Geometry: see drawing. Coordinates: mm, zero at the bounding-box minimum. Give positions to 0.01 mm unless a question says otherwise; leave off trailing zeros. Loops run counter-clockwise (first coordinate to the right, second up) from the corner with the lowest first, then second, coordinate; pieces in that order, holes last. Notation, with made-up numbers: (21.25, 67) - (70.25, 67) arc R17 ccw to (70.25, 73) - close; hole circle Ø8 at (35.5, -31). An arc over 180 degrees is marked (long way). Use one line per item in the form item = value.
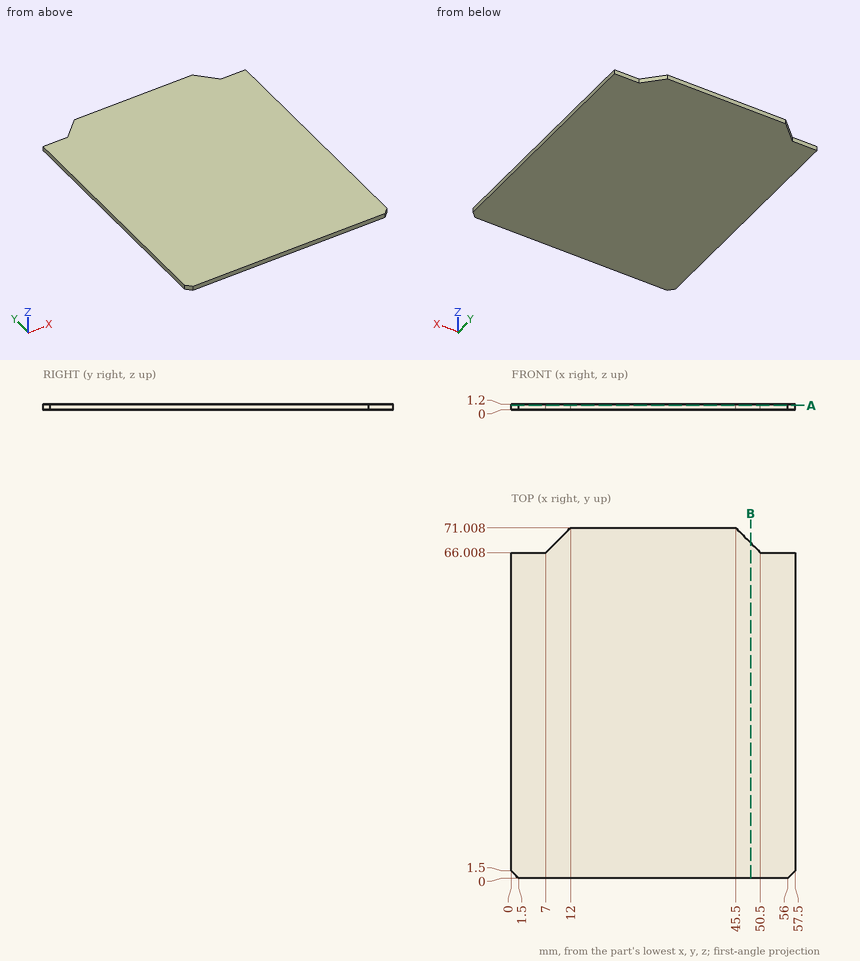
(1) Pin query (flat end, axial travel): P1, Ø0.6, axis at x = 3.5, z = 1, coming from the +Y side. Return the tip coordinate at first contact, or that it passes through.
Solution:
P1 = 66.01
(2) Material intervals for L1, parallel to Y at x = 6, z = 0.2; L2, parallel to Y at x = 11.5, z = 0.7, sorted ascending. Write a range as from..to.
Solution:
L1 = 0..66.01
L2 = 0..70.51
(3) Cut plane A-A (z = 0.9). Return the cut outline in (x, y), plus the area to 3 significant figures.
Solution:
outline = (0, 1.5) - (1.5, 0) - (56, 0) - (57.5, 1.5) - (57.5, 66.01) - (50.5, 66.01) - (45.5, 71.01) - (12, 71.01) - (7, 66.01) - (0, 66.01) - close
area = 3,990 mm2
(4) Cut plane B-B (x = 48.5). Return the cut outline in (y, z).
Solution:
outline = (0, 0) - (68.01, 0) - (68.01, 1.2) - (0, 1.2) - close
